Autodesk Inventor part; units mm, degrees
ref_plane "YZ Plane" through (0, 0, 0) normal (1, 0, 0) x (0, 1, 0)
ref_plane "XZ Plane" through (0, 0, 0) normal (0, 1, 0) x (-1, 0, 0)
ref_plane "XY Plane" through (0, 0, 0) normal (0, 0, 1) x (1, 0, 0)
sketch "Sketch1" plane through (0, 0, 0) normal (0, 0, 1) x (1, 0, 0)
  circle A0 centre (0, 0) radius 190
  circle A1 centre (0, 0) radius 300
  point P0 (0, 225)
  dimension "d41" = 600
  dimension "d42" = 380
extrude "Extrusion1" add sketch "Sketch1" along normal blind 15
sketch "Sketch3" plane through (0, 0, 0) normal (0, 0, 1) x (1, 0, 0)
  circle A0 centre (0, 0) radius 190 construction
  circle A1 centre (0, 0) radius 300 construction
  circle A2 centre (0, 0) radius 300 construction
  line L0 (0, 0) -> (0, -300) construction
  line L1 (0, 0) -> (58.5271, -294.2356) construction
  line L2 (47.602, -239.3116) -> (40.1886, -202.0418) construction
  circle A3 centre (43.8953, -220.6767) radius 7
  circle A4 centre (0, 0) radius 225 construction
  dimension "d43" = 450
  dimension "d20" = 11.25
  dimension "d21" = 14
extrude "Extrusion3" cut sketch "Sketch3" along normal through all
pattern_circular "Circular Pattern2" count 16 over 360 about axis through (0, 0, 0) along (0, 0, -1) of "Extrusion3"
equation "\"BendRadius\" = Thickness"
equation "\"BendReliefWidth\" = Thickness"
equation "\"BendReliefDepth\" = 0.5 * Thickness"
equation "\"CornerReliefSize\" = 4 * Thickness"
equation "\"MinimumRemnant\" = 2 * Thickness"
equation "\"TransitionRadius\" = BendRadius"
equation "\"JacobiRadiusSize\" = BendRadius"
equation "\"GapSize\" = Thickness"
properties part number "ДМФ 025 кольцо прижимное корма наружное v2.0"
Part model, mm, in its own coordinate system. Give positions to 0.01 mm unless a question says otherwise; leave off trailing zeros. Loops run counter-clockwise (first coordinate to the right, second up) from the corner with the lowest first, then second, coordinate; pieces in that order, holes last.
(1) Band-saw the part on D-D (x = 240.5). Write the cut outline in (y, z), and give its area (3 significant figures).
Return value:
outline: (-179.33, 0) - (179.33, 0) - (179.33, 15) - (-179.33, 15) - close
area: 5,380 mm2
(2) Drill centre lines: line 1 along Y through (x, z) = (-7, 3); line 2 along Y through (x, z) = (222.5, 8); line 3 along X through (y, z) = (217.5, 3.75). Where is each one in solid material? Low to high.
Return value:
line 1: y = -299.92 to -189.87, 189.87 to 299.92
line 2: y = -201.23 to -50.65, -37.14 to 37.14, 50.65 to 201.23
line 3: x = -206.62 to -50.13, -37.66 to 37.66, 50.13 to 206.62
(3) Band-saw the part on A-A (y = 0). Write the cut outline in (x, z).
Return value:
outline: (-300, 0) - (-190, 0) - (-190, 15) - (-300, 15) - close; (190, 0) - (300, 0) - (300, 15) - (190, 15) - close
(4) Pull direction Y, two halves, no side cores. Call faces 1 (the cylindrical face through (-39.054, -297.447, 7.395)), 2 (the cylindrical face through (122.047, -193.426, 7.395)), 3 (the flat face through (-4, -196, 15)): pulls with the +Y half, pulls with the -Y half, needs draft (parallel to the pull), parting line crosses it, or undercut.
Return value:
face 1: parting line crosses it
face 2: undercut
face 3: needs draft
(5) Band-saw the part on C-C (z = 10.5). Count the separate pieces of the cut face and the enclosed holes in it, and give its area (3 significant figures).
Return value:
separate pieces: 1
enclosed holes: 17
area: 167,000 mm2
(6) Pin check, flat tips, straight feed: pin 1 (4 mm diameter, centred on y = -200, z = 5, fed in from +X); pin 2 (3 mm diameter, centred on y = -85, z = 11, fed in from +X); pin 3 (5 mm diameter, centred on x = 94, z = 5.5, fed in from +Y). Stop position of each tip, or through.
Return value:
pin 1: stops at x = 225.38
pin 2: stops at x = 288.15
pin 3: stops at y = 285.71
